Can you work these out from the model? Positions are in its coordinate system, mm. A direction names the side the tool comes from. Give positions to 0.01 mm unless a question says otherwise; leave off trailing zeros. Loops run counter-clockwise (first coordinate to the right, second up) from the corner with the lowest first, then second, coordinate; pieces in that order, holes last. Notation, with made-up numbers: M 45,7 L 82,7 A17 ccw 82,39 Z; hole C 49.5,66 d3. An arc over 180 degrees is marked long. Put each result on its own line as item: value. Start each with the question number.
1) Imagine slicing it at C-C (z = -5). Write out the boundary of the cut face in (x, y).
2) Imagine slicing it at D-D (x = 2.75). Write out the boundary of the cut face in (y, z).
3) For P1, Ø2, axis at x = 0, z = -5, coming from the +Y side; P2, Ø1, axis at x = -1, y = 4.5, coming from the +Z side; P3, Ø7.5, axis at y = 5, z = 3.5, coming from the +X side; P4, Ø3, axis at y = 13, z = -4.5, coming from the -X side, each with a flat end and sliding along its axis, tell me the tip position at first contact or that it passes through.
4) Imagine slicing it at B-B (z = 2). Write out the boundary of the cut face in (x, y), then the cut area to 3 significant figures.
5) If we mould it in two halves opening along Y, with no side actions, what happens to faces 1 (the flat face through (3, 30, 0)), 2 (the flat face through (1, 3, 0)), 3 (the flat face through (-4, 28, 0))? For each: +Y half, -Y half, draft (parallel to the pull), parting line (faces both ways), or undercut.
6) Imagine slicing it at A-A (x = 4.75). Write out the boundary of the cut face in (y, z).
7) Please list where these lines run through material, in increasing order: line 1 along Z through (x, y) = (0, 29.2); line 2 along Y through (x, z) = (1.5, -1); line 3 along Y through (x, z) = (8.5, -1.25). Write a range as from..to.
8) For faces 4 (the cylindrical face through (-0.38, 28.03, 6.71)), 5 (the flat face through (2, 15, 0)), 6 (the flat face through (5, 0, -7.5)), which set-ups out of +Z, -Z, +X, -X, +Y, -Y let a thin tool reach every point of the face, with its end or its side?
Autodesk Inventor part; units mm, degrees
ref_plane "YZ Plane" through (0, 0, 0) normal (1, 0, 0) x (0, 1, 0)
ref_plane "XZ Plane" through (0, 0, 0) normal (0, 1, 0) x (-1, 0, 0)
ref_plane "XY Plane" through (0, 0, 0) normal (0, 0, 1) x (1, 0, 0)
sketch "Esquisse1" plane through (0, 0, 0) normal (1, 0, 0) x (0, 1, 0)
  line L0 (15, 8.5) -> (-15, 8.5)
  line L1 (-15, 8.5) -> (-15, -8.5)
  line L2 (-15, -8.5) -> (15, -8.5)
  line L3 (15, -8.5) -> (15, 8.5)
  point P0 (0, 0)
  point P1 (0, 0)
  point P2 (0, 0)
  dimension "d4" = 30
  dimension "d5" = 17
extrude "Extrusion1" add sketch "Esquisse1" along normal blind 10
sketch "Esquisse2" plane through (10, 0, 0) normal (1, 0, 0) x (0, 0, -1)
  line L0 (-7.5, 13.5) -> (7.5, 13.5)
  line L1 (7.5, 13.5) -> (7.5, -13.5)
  line L2 (7.5, -13.5) -> (-7.5, -13.5)
  line L3 (-7.5, -13.5) -> (-7.5, 13.5)
  line L4 (-7.5, 13.5) -> (7.5, -13.5)
  line L5 (-7.5, -13.5) -> (7.5, 13.5)
  point P0 (0, 0)
  point P1 (0, 0)
  point P2 (0, 0)
  dimension "d8" = 27
  dimension "d9" = 15
extrude "Extrusion2" cut sketch "Esquisse2" against normal blind 9
sketch "Esquisse3" plane through (1, 0, 0) normal (1, 0, 0) x (0, 0, -1)
  line L0 (7.5, -13.5) -> (-7.5, -13.5)
  line L1 (7.5, 13.5) -> (7.5, -13.5)
  line L2 (-7.5, -13.5) -> (7.5, -13.5)
  line L3 (7.5, -13.5) -> (7.5, -7.5)
  line L4 (7.5, -7.5) -> (-7.5, -7.5)
  line L5 (-7.5, -7.5) -> (-7.5, -13.5)
  point P0 (0, 0)
  dimension "d12" = 6
extrude "Extrusion3" cut sketch "Esquisse3" against normal blind 9
sketch "Esquisse9" plane through (0, 15, 8.5) normal (0, 1, 0) x (1, 0, 0)
  line L0 (0, 17) -> (10, 17)
  line L1 (0, 0) -> (10, 0)
  line L2 (10, 17) -> (6, 17)
  line L3 (6, 17) -> (6, 0)
  line L4 (6, 0) -> (10, 0)
  line L5 (10, 0) -> (10, 17)
  point P0 (0, 8.5)
  dimension "d58" = 4
extrude "Extrusion10" add sketch "Esquisse9" along normal blind 15
sketch "Esquisse10" plane through (6, 15, -8.5) normal (-1, 0, 0) x (0, 0, 1)
  line L0 (0, -30) -> (0, 15)
  line L1 (17, -30) -> (17, 15)
  line L2 (0, 15) -> (17, 15)
  line L3 (17, 15) -> (17, 11)
  line L4 (17, 11) -> (0, 11)
  line L5 (0, 11) -> (0, 15)
  point P0 (8.5, -15)
  point P1 (17, 15)
  point P2 (0, 11)
  dimension "d61" = 4
extrude "Extrusion11" add sketch "Esquisse10" along normal blind 10
chamfer "Chanfrein3" distance 2 angle 45 1 edges at (6, 26, 0)
chamfer "Chanfrein4" distance 2 angle 45 1 edges at (6, 15, 0)
sketch "Esquisse11" plane through (0, 30, 8.5) normal (0, 1, 0) x (1, 0, 0)
  line L0 (0, 17) -> (0, 0)
  circle A0 centre (0, 13.5) radius 1.75
  circle A1 centre (0, 3.5) radius 1.75
  line L1 (10, 17) -> (-4, 17)
  line L2 (0, 8.5) -> (10, 8.5) construction
  dimension "d70" = 3.5
  dimension "d71" = 3.5
  dimension "d72" = 10
extrude "Extrusion12" cut sketch "Esquisse11" against normal blind 10
properties part number "POUPLY_P6"
Recorded:
1. outline: M -4,26 L -1.75,26 L -1.75,30 L -4,30 Z; M 0,-15 L 10,-15 L 10,-13.5 L 0,-13.5 Z; M 0,-7.5 L 1,-7.5 L 1,13.5 L 10,13.5 L 10,30 L 1.75,30 L 1.75,26 L 4,26 L 6,24 L 6,17 L 4,15 L 0,15 Z
2. outline: M -15,-8.5 L 15,-8.5 L 15,8.5 L -15,8.5 Z; M 26,-8.5 L 30,-8.5 L 30,8.5 L 26,8.5 Z; hole M -13.5,-7.5 L 13.5,-7.5 L 13.5,7.5 L -13.5,7.5 Z
3. P1: y = 15
3. P2: through
3. P3: x = 1
3. P4: x = 0
4. outline: M -4,26 L 4,26 L 6,24 L 6,17 L 4,15 L 0,15 L 0,-7.5 L 1,-7.5 L 1,13.5 L 10,13.5 L 10,30 L -4,30 Z; M 0,-15 L 10,-15 L 10,-13.5 L 0,-13.5 Z
4. area: 155 mm²
5. face 1: +Y half
5. face 2: undercut
5. face 3: draft
6. outline: M -15,-8.5 L 15.75,-8.5 L 15.75,8.5 L -15,8.5 Z; M 25.25,-8.5 L 30,-8.5 L 30,8.5 L 25.25,8.5 Z; hole M -13.5,-7.5 L 13.5,-7.5 L 13.5,7.5 L -13.5,7.5 Z
7. line 1: -8.5..-6.75, -3.25..3.25, 6.75..8.5
7. line 2: -15..-13.5, 13.5..15, 26..30
7. line 3: -15..-13.5, 13.5..30
8. face 4: +Y
8. face 5: +Z, -Z, -X
8. face 6: +X
